Geometry: final body of the model. Coordinates: model frame, mm. Face numbers are marked on the shaded views. A direction names the side the tool comes from. Round coordinates to 2 decimals unless told otherwise and drop trailing zeros. Loops run counter-clockwise (first coordinate to the right, second up) from the corner with the lowest first, then second, coordinate; pieces in that order, holes last. Notation, with made-up numbers: (-6, 9.5) - (38, 9.5) arc R18 ccw to (38, 23.5) - close; hole circle Ø8 at (-2.75, 86). An arc over 180 degrees is marked (long way). Use CSV: the item, a comma, the result in double quotes.
from build123d import *

# Parameters (mm, degrees)
SKETCH1_R           = 5.75
SKETCH1_R_2         = 1.5
BOSS_EXTRUDE1_DEPTH = 2
CHAMFER1_SIZE       = 0.25
SKETCH2_W           = 1.75
SKETCH2_H           = 0.3


with BuildPart() as part:
    # Sketch1 → Boss-Extrude1 (new body, symmetric)
    with BuildSketch(Plane.XY):
        Circle(SKETCH1_R)
        Circle(SKETCH1_R_2, mode=Mode.SUBTRACT)
    extrude(amount=BOSS_EXTRUDE1_DEPTH, both=True)

    # Chamfer1
    chamfer1_edges = [part.edges().sort_by_distance(p)[0] for p in [
        (-5.75, 0, -2),
        (-5.75, 0, 2),
        (-1.5, 0, -2),
        (-1.5, 0, 2),
    ]]
    chamfer(chamfer1_edges, length=CHAMFER1_SIZE)

    # Sketch2 → Cut-Revolve1 (revolve, cut)
    with BuildSketch(Plane(origin=(0, 0, 0), x_dir=(1, 0, 0), z_dir=(0, 1, 0))):
        with Locations((-3.625, -1.85)):
            Rectangle(SKETCH2_W, SKETCH2_H)
    cut_revolve1 = revolve(axis=Axis((0, 0, 0), (0, 0, -1)), mode=Mode.SUBTRACT)

    # Mirror1: Cut-Revolve1 across plane
    add(cut_revolve1.mirror(Plane.XY), mode=Mode.SUBTRACT)


solid = part.part
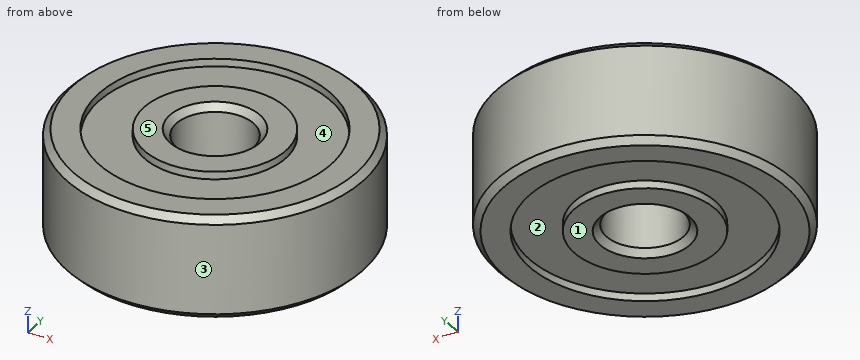
Item 1: Material intervals for line 1 (Y direction, x = 0, z = 1.85); line 2 (X direction, y = -0.5, z = -1.8); line 3 (Y direction, x = 0, z = 1.95), sorted ascending.
Final values:
line 1,"y = -5.65 to -4.5, -2.75 to -1.6, 1.6 to 2.75, 4.5 to 5.65"
line 2,"x = -5.68 to -4.47, -2.7 to -1.47, 1.47 to 2.7, 4.47 to 5.68"
line 3,"y = -5.55 to -4.5, -2.75 to -1.7, 1.7 to 2.75, 4.5 to 5.55"
Item 2: Reachability of the marked faces 1 and 2 from +Z, -Z, +X, -X, +Y, -Y: full face, straight path, thin tool, end or side. Return the list, or none.
Final values:
face 1,"-Z, +X, -X, +Y, -Y"
face 2,"-Z"
Item 3: Pin query (flat end, axial travel): P1, Ø2.5, axis at x = 0, y = 0, coming from the +Z side; P2, Ø1, axis at x = 1, z = 0, coming from the +Y side. Return the tip coordinate at first contact, or that it passes through.
Final values:
P1,"passes through"
P2,"stops at y = 5.73"
Item 4: Mould query, pull axis X, two halves, no side actions, for the marked faces 3, 4 and 5. Classes: released by +X, released by -X, zero draft, split by the parting line, or undercut.
Final values:
face 3,"split by the parting line"
face 4,"undercut"
face 5,"zero draft"
Item 5: Section B-B on z = -0.55. Return the cut outline in (x, y), plus the area to 3 significant figures.
Final values:
outline,"circle Ø11.5 at (0, 0); hole circle Ø3 at (0, 0)"
area,"96.8 mm²"
